For this review, take the finished solid that the model builds, in its own axes (mm). Round coordinates to 2 decimals unless told otherwise and drop trailing zeros. Loops run counter-clockwise (first coordinate to the right, second up) from the corner with the lowest first, then second, coordinate; pieces in that order, holes last. Notation, with made-up numbers: (8.5, 17) -> (32.5, 17) arc R6 ccw to (32.5, 24) -> close; hole circle Ø11 at (73.5, 28). An arc over 180 degrees is marked (long way). Use one line per item in the form item = value. Start each with the question number.
from build123d import *

# Parameters (mm, degrees)
F3_DEPTH = 30
F4_DEPTH = 30
F5_DEPTH = 30


with BuildPart() as f3:
    # F0 (on Front) → F3 (new body, symmetric)
    with BuildSketch(Plane.XZ):
        Polygon((-30, 12.426407), (-30, -12.426407), (-12.426407, -30), (12.426407, -30), (30, -12.426407), (30, 12.426407), (12.426407, 30), (-12.426407, 30), align=None)
    extrude(amount=F3_DEPTH, both=True)

    # F1 (on Top) → F4 (intersect, symmetric)
    with BuildSketch(Plane.XY):
        Polygon((30, -12.426407), (30, 12.426407), (12.426407, 30), (-12.426407, 30), (-30, 12.426407), (-30, -12.426407), (-12.426407, -30), (12.426407, -30), align=None)
    extrude(amount=F4_DEPTH, both=True, mode=Mode.INTERSECT)

    # F2 (on Right) → F5 (intersect, symmetric)
    with BuildSketch(Plane.YZ):
        Polygon((12.426407, 30), (-12.426407, 30), (-30, 12.426407), (-30, -12.426407), (-12.426407, -30), (12.426407, -30), (30, -12.426407), (30, 12.426407), align=None)
    extrude(amount=F5_DEPTH, both=True, mode=Mode.INTERSECT)


solid = f3.part
Item 1: Take a section at A-A on y = -7. Give the boundary of the cut face in (x, z), plus the area to 3 significant figures.
Item 2: For P1, Ø2, axis at y = 20.5, z = 11, coming from the +X side; P2, Ø6, axis at y = 8.5, z = -23, coming from the -X side; P3, Ø3, axis at y = -2, z = -16, coming from the -X side, all flat-tipped, find the tip position at first contact; note any pin that passes through.
Item 3: Take a section at D-D on z = -25.5. Give the boundary of the cut face in (x, y), plus the area to 3 significant figures.
Item 4: Take a section at C-C on x = -23. Give the boundary of the cut face in (y, z).
Item 5: Wall thickness on line 1 (Z direction, x = 14, y = 10); line 2 (X direction, y = 21, z = -12.5); line 3 (Z direction, x = 2, y = 24): over which ranges is each line inside the solid? List them lowest first.
Results:
q1.outline = (-30, -12.43) -> (-12.43, -30) -> (12.43, -30) -> (30, -12.43) -> (30, 12.43) -> (12.43, 30) -> (-12.43, 30) -> (-30, 12.43) -> close
q1.area = 2,980 mm2
q2.P1 = 22.93
q2.P2 = -22.43
q2.P3 = -27.93
q3.outline = (-16.93, -16.93) -> (16.93, -16.93) -> (16.93, 16.93) -> (-16.93, 16.93) -> close
q3.area = 1,150 mm2
q4.outline = (-19.43, -19.43) -> (19.43, -19.43) -> (19.43, 19.43) -> (-19.43, 19.43) -> close
q5.line_1 = -28.43 to 28.43
q5.line_2 = -21.43 to 21.43
q5.line_3 = -18.43 to 18.43
